from build123d import *

# Parameters (mm, degrees)
SZKIC1_R                    = 4.5
DODANIE_WYCI_GNI_CIE1_DEPTH = 200


with BuildPart() as part:
    # Szkic1 → Dodanie-wyciągnięcie1 (new body)
    with BuildSketch(Plane.XY):
        with BuildLine():
            Line((4, 7.75478035), (-4, 7.75478035))
            ThreePointArc((-4, 7.75478035), (-7.445030717, 10.96569241), (-8.717134168, 15.500000044))
            ThreePointArc((-8.717134168, 15.500000044), (-8.058124425, 17.090990301), (-6.467134168, 17.750000044))
            Line((-6.467134168, 17.750000044), (-6.467134168, 15.500000044))
            Line((-6.467134168, 15.500000044), (-4, 15.500000044))
            Line((-4, 15.500000044), (-4, 20.000000044))
            Line((-4, 20.000000044), (-19, 20.000000044))
            ThreePointArc((-19, 20.000000044), (-19.707106812, 19.707106812), (-20.000000044, 19))
            Line((-20.000000044, 19), (-20.000000044, 4))
            Line((-20.000000044, 4), (-15.500000044, 4))
            Line((-15.500000044, 4), (-15.500000044, 6.471381771))
            Line((-15.500000044, 6.471381771), (-17.750000044, 6.471381771))
            ThreePointArc((-17.750000044, 6.471381771), (-17.090990301, 8.062372029), (-15.500000044, 8.721381771))
            ThreePointArc((-15.500000044, 8.721381771), (-10.962546302, 7.448087912), (-7.750000044, 4))
            Line((-7.750000044, 4), (-7.750000044, -4))
            ThreePointArc((-7.750000044, -4), (-10.962546302, -7.448087912), (-15.500000044, -8.721381771))
            ThreePointArc((-15.500000044, -8.721381771), (-17.090990301, -8.062372029), (-17.750000044, -6.471381771))
            Line((-17.750000044, -6.471381771), (-15.500000044, -6.471381771))
            Line((-15.500000044, -6.471381771), (-15.500000044, -4))
            Line((-15.500000044, -4), (-20.000000044, -4))
            Line((-20.000000044, -4), (-20.000000044, -19))
            ThreePointArc((-20.000000044, -19), (-19.707106812, -19.707106812), (-19, -20.000000044))
            Line((-19, -20.000000044), (-4, -20.000000044))
            Line((-4, -20.000000044), (-4, -15.500000044))
            Line((-4, -15.500000044), (-6.467134168, -15.500000044))
            Line((-6.467134168, -15.500000044), (-6.467134168, -17.750000044))
            ThreePointArc((-6.467134168, -17.750000044), (-8.058124425, -17.090990301), (-8.717134168, -15.500000044))
            ThreePointArc((-8.717134168, -15.500000044), (-7.445030717, -10.96569241), (-4, -7.75478035))
            Line((-4, -7.75478035), (4, -7.75478035))
            ThreePointArc((4, -7.75478035), (7.445030717, -10.96569241), (8.717134168, -15.500000044))
            ThreePointArc((8.717134168, -15.500000044), (8.058124425, -17.090990301), (6.467134168, -17.750000044))
            Line((6.467134168, -17.750000044), (6.467134168, -15.500000044))
            Line((6.467134168, -15.500000044), (4, -15.500000044))
            Line((4, -15.500000044), (4, -20.000000044))
            Line((4, -20.000000044), (19, -20.000000044))
            ThreePointArc((19, -20.000000044), (19.707106812, -19.707106812), (20.000000044, -19))
            Line((20.000000044, -19), (20.000000044, -4))
            Line((20.000000044, -4), (15.500000044, -4))
            Line((15.500000044, -4), (15.500000044, -6.471381771))
            Line((15.500000044, -6.471381771), (17.750000044, -6.471381771))
            ThreePointArc((17.750000044, -6.471381771), (17.090990301, -8.062372029), (15.500000044, -8.721381771))
            ThreePointArc((15.500000044, -8.721381771), (10.962546302, -7.448087912), (7.750000044, -4))
            Line((7.750000044, -4), (7.750000044, 4))
            ThreePointArc((7.750000044, 4), (10.962546302, 7.448087912), (15.500000044, 8.721381771))
            ThreePointArc((15.500000044, 8.721381771), (17.090990301, 8.062372029), (17.750000044, 6.471381771))
            Line((17.750000044, 6.471381771), (15.500000044, 6.471381771))
            Line((15.500000044, 6.471381771), (15.500000044, 4))
            Line((15.500000044, 4), (20.000000044, 4))
            Line((20.000000044, 4), (20.000000044, 19))
            ThreePointArc((20.000000044, 19), (19.707106812, 19.707106812), (19, 20.000000044))
            Line((19, 20.000000044), (4, 20.000000044))
            Line((4, 20.000000044), (4, 15.500000044))
            Line((4, 15.500000044), (6.467134168, 15.500000044))
            Line((6.467134168, 15.500000044), (6.467134168, 17.750000044))
            ThreePointArc((6.467134168, 17.750000044), (8.058124425, 17.090990301), (8.717134168, 15.500000044))
            ThreePointArc((8.717134168, 15.500000044), (7.445030717, 10.96569241), (4, 7.75478035))
        make_face()
        Circle(SZKIC1_R, mode=Mode.SUBTRACT)
        with BuildLine():
            Line((-17.750000044, 10.971381771), (-17.750000044, 16.754247647))
            ThreePointArc((-17.750000044, 16.754247647), (-17.457106825, 17.461354428), (-16.750000044, 17.754247647))
            Line((-16.750000044, 17.754247647), (-10.967134168, 17.754247647))
            Line((-10.967134168, 17.754247647), (-10.967134168, 10.971381771))
            Line((-10.967134168, 10.971381771), (-17.750000044, 10.971381771))
        make_face(mode=Mode.SUBTRACT)
        with BuildLine():
            Line((10.967134168, 10.971381771), (17.750000044, 10.971381771))
            Line((17.750000044, 10.971381771), (17.750000044, 16.754247647))
            ThreePointArc((17.750000044, 16.754247647), (17.457106825, 17.461354428), (16.750000044, 17.754247647))
            Line((16.750000044, 17.754247647), (10.967134168, 17.754247647))
            Line((10.967134168, 17.754247647), (10.967134168, 10.971381771))
        make_face(mode=Mode.SUBTRACT)
        with BuildLine():
            Line((17.750000044, -10.971381771), (17.750000044, -16.754247647))
            ThreePointArc((17.750000044, -16.754247647), (17.457106825, -17.461354428), (16.750000044, -17.754247647))
            Line((16.750000044, -17.754247647), (10.967134168, -17.754247647))
            Line((10.967134168, -17.754247647), (10.967134168, -10.971381771))
            Line((10.967134168, -10.971381771), (17.750000044, -10.971381771))
        make_face(mode=Mode.SUBTRACT)
        with BuildLine():
            Line((-10.967134168, -10.971381771), (-17.750000044, -10.971381771))
            Line((-17.750000044, -10.971381771), (-17.750000044, -16.754247647))
            ThreePointArc((-17.750000044, -16.754247647), (-17.457106825, -17.461354428), (-16.750000044, -17.754247647))
            Line((-16.750000044, -17.754247647), (-10.967134168, -17.754247647))
            Line((-10.967134168, -17.754247647), (-10.967134168, -10.971381771))
        make_face(mode=Mode.SUBTRACT)
    extrude(amount=DODANIE_WYCI_GNI_CIE1_DEPTH)


solid = part.part
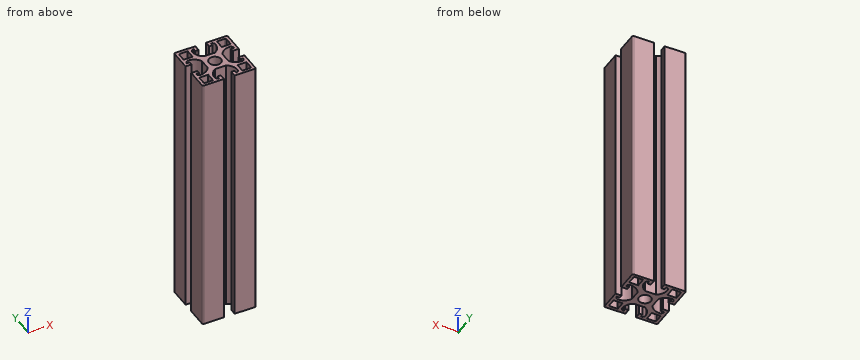
Source: CAD feature listing. Evaluate the final solid. Frame: model axes, mm. Give positions to 0.01 mm unless a question says otherwise; leave off trailing zeros. Write each loop counter-clockwise with the first axis right and the second up, starting at its lowest first coordinate (ties: lowest second). Pieces come first, ordered by that corner, then holes. Notation, with made-up numbers: M 18,-3.5 L 38,-3.5 A10 ccw 38,5.5 Z; hole C 50,36 d4. An arc over 180 degrees is marked long. Return JSON: item names as keys, results as strings. Group by question number.
1) Cut plane D-D, the plane y = -13. Output: boundary loops of the cut face in (x, z).
2) Cut plane A-A, the plane y = 0. Output: boundary loops of the cut face in (x, z).
3) First-contact query: pin 1 Ø1.5 at (x, y) = (9, -8) entering from -Z. Flat tip, straight axial feed; report the tip coordinate or a pass-through.
4) Ray query, L1, parallel to Y at x = -5, z = 117.5; L2, parallel to X at y = -12, z = 76.5; L3, parallel to X at y = 11.5, z = 105. Return the intervals inside material, ascending.
5) Cut plane C-C, the plane z = 161. Give the number of separate pieces and of enclosed holes in the cut face, then the cut area to 3 significant figures.
Data:
{
 "1": {"outline": "M -20,0 L -17.75,0 L -17.75,200 L -20,200 Z; M -10.97,0 L -8.35,0 L -8.35,200 L -10.97,200 Z; M 8.35,0 L 10.97,0 L 10.97,200 L 8.35,200 Z; M 17.75,0 L 20,0 L 20,200 L 17.75,200 Z"},
 "2": {"outline": "M -7.75,0 L -4.5,0 L -4.5,200 L -7.75,200 Z; M 4.5,0 L 7.75,0 L 7.75,200 L 4.5,200 Z"},
 "3": {"pin 1": "stops at z = 0"},
 "4": {"L1": "y = -20 to -15.5, -8.36 to 8.36, 15.5 to 20", "L2": "x = -20 to -17.75, -10.97 to -7.98, 7.98 to 10.97, 17.75 to 20", "L3": "x = -20 to -17.75, -10.97 to -7.75, 7.75 to 10.97, 17.75 to 20"},
 "5": {"separate pieces": "1", "enclosed holes": "5", "area": "720 mm²"}
}
